For this review, take the finished solid that the model builds, in its own axes (mm). A direction names the side the tool comes from. Round coordinates to 2 decimals unless told otherwise and drop trailing zeros. Order: outer loops, then holes, each group sorted by start corner. A loop starts at its lowest first (then second) coordinate and runs counter-clockwise, first axis right, second up. Notation, with made-up numbers: M -25.5,23.5 L 22.5,23.5 A11 ccw 22.5,42.5 Z; hole C -1.5,18.5 d6. An arc over 180 degrees is marked long. Put each result on its own line as item: value.
from build123d import *

# Parameters (mm, degrees)
EXTRUDE_1_DEPTH                 = 20
SKETCH_2_R                      = 1.65
CUT_EXTRUDE_1_DEPTH             = 4
CUT_EXTRUDE_1_DIRECTION_2_REACH = 31.954
CUT_EXTRUDE_START               = -21
SKETCH_3_R                      = 3
CUT_EXTRUDE_2_DEPTH             = 21
SKETCH_4_R                      = 1.65
CUT_EXTRUDE_3_DEPTH             = 4
CUT_EXTRUDE_3_DIRECTION_2_REACH = 34.265
CUT_EXTRUDE_7_REACH             = 34.265
SKETCH_5_R                      = 3
CUT_EXTRUDE_8_DEPTH             = 21
FILLET_1_R                      = 10
FILLET_2_R                      = 1


with BuildPart() as part:
    # Эскиз1 → Бобышка-Вытянуть1 (new body)
    with BuildSketch(Plane(origin=(0, 0, 0), x_dir=(0, 0, -1), z_dir=(1, 0, 0))):
        Polygon((0, 0), (7.5, 0), (7.5, 4), (4, 25), (0, 25), align=None)
    extrude(amount=EXTRUDE_1_DEPTH)

    # Эскиз2 → Вырез-Вытянуть1 (cut)
    with BuildSketch(Plane(origin=(0, 4, 0), x_dir=(-1, 0, 0), z_dir=(0, -1, 0))):
        with Locations(Location((-16.5, 4.25, 0), (0, 0, 270))):
            Circle(SKETCH_2_R)
        with Locations(Location((-3.5, 4.25, 0), (0, 0, 270))):
            Circle(SKETCH_2_R)
    extrude(amount=CUT_EXTRUDE_1_DEPTH, mode=Mode.SUBTRACT)

    # Вырез-Вытянуть1 direction 2: up to this plane
    cut_extrude_1_direction_2_end = Plane(origin=(20, 25, -4), z_dir=(0, -0.16439898730535726, 0.9863939238321437))
    # Эскиз2 → Вырез-Вытянуть1 direction 2 (cut, up to the surface)
    with BuildSketch(Plane(origin=(0, 4, 0), x_dir=(-1, 0, 0), z_dir=(0, -1, 0)), mode=Mode.PRIVATE) as cut_extrude_1_direction_2_sk1:
        with Locations(Location((-16.5, 4.25, 0), (0, 0, 270))):
            Circle(SKETCH_2_R)
    cut_extrude_1_direction_2_tool1 = split(extrude(cut_extrude_1_direction_2_sk1.sketch, amount=-CUT_EXTRUDE_1_DIRECTION_2_REACH, mode=Mode.PRIVATE), bisect_by=cut_extrude_1_direction_2_end, keep=Keep.BOTH, mode=Mode.PRIVATE)
    add(cut_extrude_1_direction_2_tool1.solids().sort_by_distance((16.5, 4, -4.25))[0], mode=Mode.SUBTRACT)
    # Эскиз2 → Вырез-Вытянуть1 direction 2 (cut, up to the surface)
    with BuildSketch(Plane(origin=(0, 4, 0), x_dir=(-1, 0, 0), z_dir=(0, -1, 0)), mode=Mode.PRIVATE) as cut_extrude_1_direction_2_sk2:
        with Locations(Location((-3.5, 4.25, 0), (0, 0, 270))):
            Circle(SKETCH_2_R)
    cut_extrude_1_direction_2_tool2 = split(extrude(cut_extrude_1_direction_2_sk2.sketch, amount=-CUT_EXTRUDE_1_DIRECTION_2_REACH, mode=Mode.PRIVATE), bisect_by=cut_extrude_1_direction_2_end, keep=Keep.BOTH, mode=Mode.PRIVATE)
    add(cut_extrude_1_direction_2_tool2.solids().sort_by_distance((3.5, 4, -4.25))[0], mode=Mode.SUBTRACT)

    # Эскиз3 → Вырез-Вытянуть2 (cut)
    with BuildSketch(Plane(origin=(0, 4, 0), x_dir=(-1, 0, 0), z_dir=(0, -1, 0)).offset(CUT_EXTRUDE_START)):
        with Locations(Location((-16.5, 4.25, 0), (0, 0, 90))):
            Circle(SKETCH_3_R)
        with Locations(Location((-3.5, 4.25, 0), (0, 0, 90))):
            Circle(SKETCH_3_R)
    extrude(amount=CUT_EXTRUDE_2_DEPTH, mode=Mode.SUBTRACT)

    # Эскиз4 → Вырез-Вытянуть3 (cut)
    with BuildSketch(Plane.XY.offset(-4)):
        with Locations(Location((10, 21.35, 0), (0, 0, 180))):
            Circle(SKETCH_4_R)
        with Locations(Location((10, 9.35, 0), (0, 0, 180))):
            Circle(SKETCH_4_R)
    extrude(amount=CUT_EXTRUDE_3_DEPTH, mode=Mode.SUBTRACT)

    # Вырез-Вытянуть3 direction 2: up to this plane
    cut_extrude_3_direction_2_end = Plane(origin=(20, 25, -4), z_dir=(0, -0.16439898730535726, 0.9863939238321437))
    # Эскиз4 → Вырез-Вытянуть3 direction 2 (cut, up to the surface)
    with BuildSketch(Plane.XY.offset(-4), mode=Mode.PRIVATE) as cut_extrude_3_direction_2_sk1:
        with Locations(Location((10, 21.35, 0), (0, 0, 180))):
            Circle(SKETCH_4_R)
    cut_extrude_3_direction_2_tool1 = split(extrude(cut_extrude_3_direction_2_sk1.sketch, amount=-CUT_EXTRUDE_3_DIRECTION_2_REACH, mode=Mode.PRIVATE), bisect_by=cut_extrude_3_direction_2_end, keep=Keep.BOTH, mode=Mode.PRIVATE)
    add(cut_extrude_3_direction_2_tool1.solids().sort_by_distance((10, 21.35, -4))[0], mode=Mode.SUBTRACT)
    # Эскиз4 → Вырез-Вытянуть3 direction 2 (cut, up to the surface)
    with BuildSketch(Plane.XY.offset(-4), mode=Mode.PRIVATE) as cut_extrude_3_direction_2_sk2:
        with Locations(Location((10, 9.35, 0), (0, 0, 180))):
            Circle(SKETCH_4_R)
    cut_extrude_3_direction_2_tool2 = split(extrude(cut_extrude_3_direction_2_sk2.sketch, amount=-CUT_EXTRUDE_3_DIRECTION_2_REACH, mode=Mode.PRIVATE), bisect_by=cut_extrude_3_direction_2_end, keep=Keep.BOTH, mode=Mode.PRIVATE)
    add(cut_extrude_3_direction_2_tool2.solids().sort_by_distance((10, 9.35, -4))[0], mode=Mode.SUBTRACT)

    # Вырез-Вытянуть7: up to this plane
    cut_extrude_7_end = Plane(origin=(20, 25, -4), z_dir=(0, -0.16439898730535726, 0.9863939238321437))
    # Эскиз5 → Вырез-Вытянуть7 (cut, up to the surface)
    with BuildSketch(Plane.XY.offset(-4), mode=Mode.PRIVATE) as cut_extrude_7_sk1:
        with Locations((10, 21.35)):
            Circle(SKETCH_5_R)
    cut_extrude_7_tool1 = split(extrude(cut_extrude_7_sk1.sketch, amount=-CUT_EXTRUDE_7_REACH, mode=Mode.PRIVATE), bisect_by=cut_extrude_7_end, keep=Keep.BOTH, mode=Mode.PRIVATE)
    add(cut_extrude_7_tool1.solids().sort_by_distance((10, 21.35, -4))[0], mode=Mode.SUBTRACT)
    # Эскиз5 → Вырез-Вытянуть7 (cut, up to the surface)
    with BuildSketch(Plane.XY.offset(-4), mode=Mode.PRIVATE) as cut_extrude_7_sk2:
        with Locations((10, 9.35)):
            Circle(SKETCH_5_R)
    cut_extrude_7_tool2 = split(extrude(cut_extrude_7_sk2.sketch, amount=-CUT_EXTRUDE_7_REACH, mode=Mode.PRIVATE), bisect_by=cut_extrude_7_end, keep=Keep.BOTH, mode=Mode.PRIVATE)
    add(cut_extrude_7_tool2.solids().sort_by_distance((10, 9.35, -4))[0], mode=Mode.SUBTRACT)

    # Эскиз6 → Вырез-Вытянуть8 (cut)
    with BuildSketch(Plane(origin=(0, 25, 0), x_dir=(1, 0, 0), z_dir=(0, 1, 0))):
        Polygon((0, 7.5), (0, 1.25), (3.5, 1.25), (3.5, 4.25), (6.5, 4.25), (6.5, 7.5), align=None)
        Polygon((13.5, 4.25), (16.5, 4.25), (16.5, 1.25), (20, 1.25), (20, 7.5), (13.5, 7.5), align=None)
    extrude(amount=-CUT_EXTRUDE_8_DEPTH, mode=Mode.SUBTRACT)

    # Скругление1
    fillet_1_edges = [part.edges().sort_by_distance(p)[0] for p in [
        (0, 25, -0.625),
        (20, 25, -0.625),
    ]]
    fillet(fillet_1_edges, radius=FILLET_1_R - 0.0001)  # a hair under: the kernel refuses the full size

    # Скругление2
    fillet_2_edges = [part.edges().sort_by_distance(p)[0] for p in [
        (20, 2, -7.5),
        (0, 2, -7.5),
    ]]
    fillet(fillet_2_edges, radius=FILLET_2_R)


solid = part.part
(1) Draft analysis for pull direction Y (two halves, no side actions). For faces 5 (the face through (10, 0, -4)), 6 (the face through (20, 4, -1)), 7 (the face through (11.3, 8.1, -4)), state which applies: released by +Y, released by -Y, zero draft, split by the parting line, or undercut.
A:
face 5: released by -Y
face 6: zero draft
face 7: undercut
(2) Add section C-C on y = 1.5. Give the boundary of the cut face in (x, z), then the cut area to 3 significant figures.
A:
outline: M 0,-6.5 A1 ccw 1,-7.5 L 19,-7.5 A1 ccw 20,-6.5 L 20,0 L 0,0 Z; hole C 3.5,-4.25 d3.3; hole C 16.5,-4.25 d3.3
area: 132 mm2
(3) Add section B-B on y = 21.35. Give the boundary of the cut face in (x, z).
A:
outline: M 2.27,-1.25 L 3.5,-1.25 A3 cw 6.5,-4.25 L 6.5,-4.61 L 7,-4.61 L 7,-4 L 8.35,-4 L 8.35,0 L 2.27,0 Z; M 11.65,-4 L 13,-4 L 13,-4.61 L 13.5,-4.61 L 13.5,-4.25 A3 cw 16.5,-1.25 L 17.73,-1.25 L 17.73,0 L 11.65,0 Z
(4) To check wall thickness, follow L1, parallel to Y at x = 10, z = -2.3; L2, parallel to X at y = 2.55, z = -4.25; L3, parallel to Z at x = 16.5, y = 0.8. State the ranges of each line that lie inside material, in increasing order.
A:
L1: y = 0 to 7.7, 11 to 19.7, 23 to 25
L2: x = 0 to 1.85, 5.15 to 14.85, 18.15 to 20
L3: z = -7.5 to -5.9, -2.6 to 0
(5) Insertion check: pin 1 Ø3 at (x, y) = (18.5, 14) entering from -Z; pin 2 Ø6.5 at (x, y) = (10.5, 9) entering from -Z; pin 3 Ø3 at (x, z) = (3.5, -6) entering from +Y. Each pin has a flat end and moves straight along its axis. Give the tip position at first contact, or say it passes through.
A:
pin 1: stops at z = -1.25
pin 2: stops at z = -7.21
pin 3: stops at y = 4
(6) Add section A-A on z = -5.5. Give the boundary of the cut face in (x, y).
A:
outline: M 0,0 L 2.42,0 L 2.42,4 L 0,4 Z; M 4.58,0 L 15.42,0 L 15.42,4 L 13.5,4 L 13.5,16 L 6.5,16 L 6.5,4 L 4.58,4 Z; M 17.58,0 L 20,0 L 20,4 L 17.58,4 Z; hole C 10,9.35 d6
(7) Add section D-D on z = -3.25. State how many separate pieces and enclosed holes the cut face has, then the cut area to 3 significant figures.
A:
separate pieces: 3
enclosed holes: 2
area: 194 mm2
(8) For faces 1 (the face through (18, 11, -1.25)), 2 (the face through (9.951, 14.353, -5.774)), 3 (the face through (6.5, 10, -5)), 4 (the face through (11.384, 6.688, -5.226)), list the 3-axis set-ups (+Z, -Z, +X, -X, +Y, -Y) from which the entire face can be reached by the end or side of a thin tool; tool diameter is ignored.
A:
face 1: -Z, +X, +Y
face 2: -Z, +X, -X, +Y
face 3: -Z, -X, +Y
face 4: -Z
